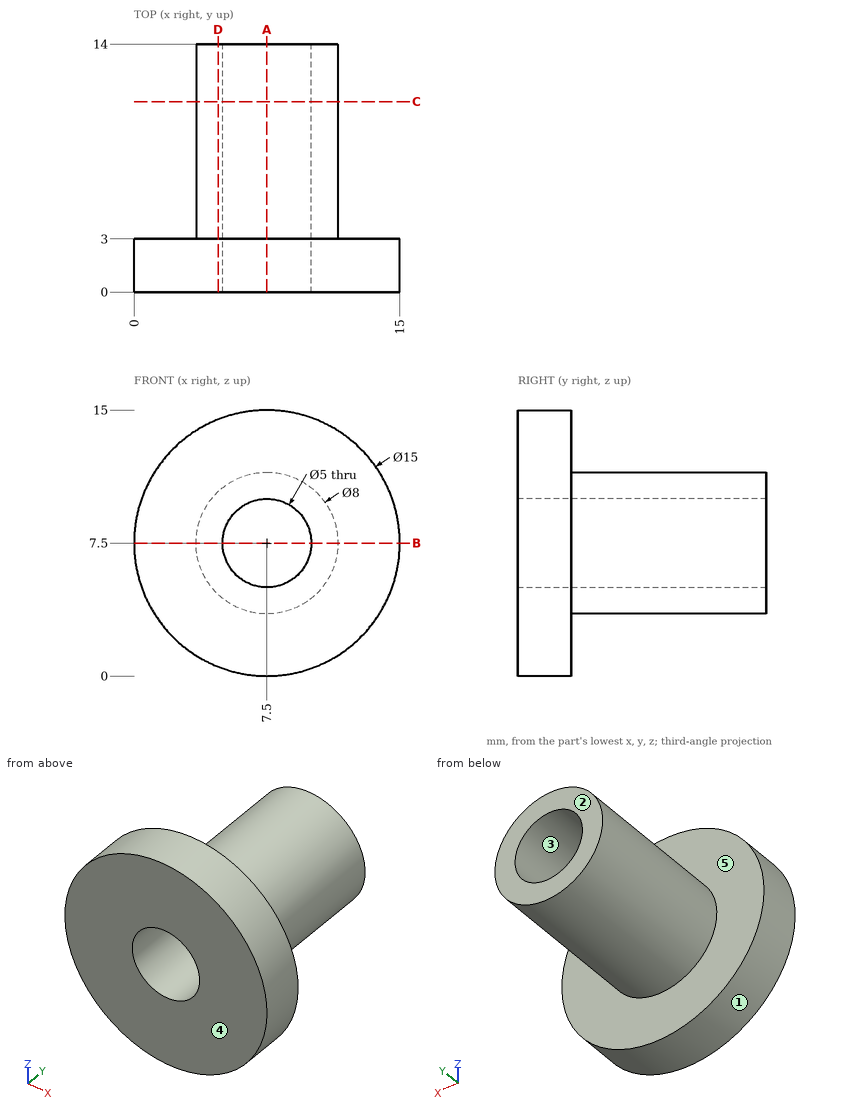
Answer from the drawing. Dimensions are ordinates in mm from the lowest x, y and z of the part. A direction names the side the tool comes from. Give positions to 0.01 mm unless a question says otherwise; leave off trailing zeros. Order: outer loops, then holes, each group sorted by start corner. A loop starts at its lowest first (then second) coordinate and runs counter-clockwise, first axis right, second up. Notation, with made-up numbers: (-35, -17) -> (-1, -17) arc R30 ccw to (-1, 8) -> close; hole circle Ø8 at (-14.75, 77.5). An arc over 180 degrees is marked (long way). One line per item, written item: value.
Item 1: Find section A-A, the plane x = 7.5. Give the vertices of the cut face in (y, z), plus the area to 3 significant figures.
Answer sheet:
outline: (0, 0) -> (3, 0) -> (3, 3.5) -> (14, 3.5) -> (14, 5) -> (0, 5) -> close; (0, 10) -> (14, 10) -> (14, 11.5) -> (3, 11.5) -> (3, 15) -> (0, 15) -> close
area: 63.0 mm²
Item 2: Find section D-D, the plane x = 4.75. Give the vertices of the cut face in (y, z), plus the area to 3 significant figures.
Answer sheet:
outline: (0, 0.52) -> (3, 0.52) -> (3, 4.6) -> (14, 4.6) -> (14, 10.4) -> (3, 10.4) -> (3, 14.48) -> (0, 14.48) -> close
area: 106 mm²
Item 3: Find section C-C, the plane y = 10.75. Give the vertices of the cut face in (x, z).
Answer sheet:
outline: circle Ø8 at (7.5, 7.5); hole circle Ø5 at (7.5, 7.5)
Item 4: Find section B-B, the plane z = 7.5. Give the vertices of the cut face in (x, y).
Answer sheet:
outline: (0, 0) -> (5, 0) -> (5, 14) -> (3.5, 14) -> (3.5, 3) -> (0, 3) -> close; (10, 0) -> (15, 0) -> (15, 3) -> (11.5, 3) -> (11.5, 14) -> (10, 14) -> close
Item 5: A tool of negligible diameter and unlimited length cuts with its end or side. For the marked faces 4 and 5, from which of +Z, -Z, +X, -X, +Y, -Y can it reach the whole face along a straight path? Write none if from no direction.
Answer sheet:
face 4: +Z, -Z, +X, -X, -Y
face 5: +Y
Item 6: Determine the mould class of the marked faces 1, 2 and 3 for opening direction Z: released by +Z, released by -Z, zero draft, split by the parting line, or undercut.
Answer sheet:
face 1: split by the parting line
face 2: zero draft
face 3: undercut
Item 7: Flat-ended cylindrical pins translate along their axes: P1, Ø1.5, axis at x = 9.5, y = 7, coming from the -Z side; P2, Ø1, axis at x = 7, y = 10.5, coming from the -Z side; P3, Ø6, axis at x = 12, y = 6.5, coming from the -Z side. Find the tip coordinate at first contact, or state that the pin passes through.
Answer sheet:
P1: z = 3.7
P2: z = 3.5
P3: z = 3.79
Item 8: Straight lines are drawn through the part: probe 1 along X at (y, z) = (3.5, 7.5); probe 2 along Y at (x, z) = (12, 8.5); probe 3 along X at (y, z) = (3.25, 6.25). For each, find the intervals that lie inside material, in ascending order.
Answer sheet:
probe 1: 3.5 to 5, 10 to 11.5
probe 2: 0 to 3
probe 3: 3.7 to 5.33, 9.67 to 11.3
